Model file for the job. Use its own axes, mm. A direction names the side the tool comes from. Give positions to 0.01 mm unless a question says otherwise; leave off trailing zeros. Write each loop counter-clockwise with the first axis right and the second up, starting at its lowest first coordinate (ties: lowest second). Pieces come first, ordered by that corner, then holes. Notation, with made-up numbers: (5, 7) - (36, 7) arc R24 cw to (36, 17) - close; hole circle Ø11 at (74.5, 46). An arc over 180 degrees is marked (long way). Use CSV: the item, a comma, the result in double quotes.
from build123d import *

# Parameters (mm, degrees)
SKETCH1_R               = 61.9125
BASE_EXTRUDE_DEPTH      = 7.9248
BASE_EXTRUDE_DEPTH_BACK = 33.6677
SKETCH11_R              = 33.3375
CUT_EXTRUDE1_DEPTH      = 9.525
SKETCH12_R              = 35.7124
CUT_EXTRUDE2_DEPTH      = 2.5748
CUT_EXTRUDE2_DEPTH_BACK = 4.7752
SKETCH13_R              = 12.7
CUT_EXTRUDE3_DEPTH      = 41.0177
SKETCH32_R              = 6.7437
CUT_EXTRUDE4_DEPTH      = 45.72


with BuildPart() as part:
    # Sketch1 → Base-Extrude (new body, two sides)
    with BuildSketch(Plane(origin=(0, 0, 0), x_dir=(1, 0, 0), z_dir=(0, 1, 0))) as base_extrude_sk:
        with Locations(Location((0, 0, 0), (0, 0, 270))):  # turned: the seam where the file's is
            Circle(SKETCH1_R)
    extrude(amount=BASE_EXTRUDE_DEPTH)
    extrude(base_extrude_sk.sketch, amount=-BASE_EXTRUDE_DEPTH_BACK)

    # Sketch11 → Cut-Extrude1 (cut)
    with BuildSketch(Plane(origin=(0, 6.35, 0), x_dir=(-1, 0, 0), z_dir=(0, 1, 0))):
        with Locations(Location((0, 0, 0), (0, 0, 90))):  # turned: the seam where the file's is
            Circle(SKETCH11_R)
    extrude(amount=-CUT_EXTRUDE1_DEPTH, mode=Mode.SUBTRACT)

    # Sketch12 → Cut-Extrude2 (cut, two sides)
    with BuildSketch(Plane(origin=(0, 6.35, 0), x_dir=(-1, 0, 0), z_dir=(0, 1, 0))) as cut_extrude2_sk:
        with Locations(Location((0, 0, 0), (0, 0, 90))):  # turned: the seam where the file's is
            Circle(SKETCH12_R)
    extrude(amount=CUT_EXTRUDE2_DEPTH, mode=Mode.SUBTRACT)
    extrude(cut_extrude2_sk.sketch, amount=-CUT_EXTRUDE2_DEPTH_BACK, mode=Mode.SUBTRACT)

    # Sketch13 → Cut-Extrude3 (cut, through all)
    with BuildSketch(Plane(origin=(0, 6.35, 0), x_dir=(-1, 0, 0), z_dir=(0, 1, 0))):
        with Locations(Location((0, 0, 0), (0, 0, 90))):  # turned: the seam where the file's is
            Circle(SKETCH13_R)
    extrude(amount=-CUT_EXTRUDE3_DEPTH, mode=Mode.SUBTRACT)

    # Sketch32 → Cut-Extrude4 (cut)
    with BuildSketch(Plane(origin=(0, 7.9248, 0), x_dir=(-1, 0, 0), z_dir=(0, 1, 0))):
        with Locations(Location((0, -50.8, 0), (0, 0, 90))):  # turned: the seam where the file's is
            Circle(SKETCH32_R)
        with Locations(Location((-43.994090512, 25.4, 0), (0, 0, 90))):  # turned: the seam where the file's is
            Circle(SKETCH32_R)
        with Locations(Location((43.994090512, 25.4, 0), (0, 0, 90))):  # turned: the seam where the file's is
            Circle(SKETCH32_R)
    extrude(amount=-CUT_EXTRUDE4_DEPTH, mode=Mode.SUBTRACT)


solid = part.part
(1) Saw through at D-D, the plane y = 5. List the corners of the cut face in (x, z) (1 decimal), then the cut area to 3 significant figures.
Checked values:
outline,"circle Ø123.8 at (0, 0); hole circle Ø13.5 at (-44, 25.4); hole circle Ø71.4 at (0, 0); hole circle Ø13.5 at (0, -50.8); hole circle Ø13.5 at (44, 25.4)"
area,"7,610 mm^2"
(2) Pull direction X, two halves, no side cores. Call faces 1 (the face through (10.727, 4.705, 34.063)), 2 (the face through (1, -33.668, 13)), 3 (the face through (-60.44, -12.58, -13.42)): released by +X, released by -X, zero draft, split by the parting line, or undercut.
Checked values:
face 1,"undercut"
face 2,"zero draft"
face 3,"split by the parting line"
(3) Wall check: probe 1 along X at (y, z) = (-8, 25); probe 2 along Z at (x, y) = (-5, -17.5); probe 3 along X at (y, z) = (-16, 0). Give the ranges that are in metal, low to high. Write a range as [from, to].
Checked values:
probe 1,"x = [-56.64, -50.73], [-37.26, 37.26], [50.73, 56.64]"
probe 2,"z = [-61.71, -55.33], [-46.27, -11.67], [11.67, 61.71]"
probe 3,"x = [-61.91, -12.7], [12.7, 61.91]"
(4) Saw through at C-C, the plane z = 25.4. List the corners of the cut face in (x, y) (3 decimals).
Checked values:
outline,"(-56.462, -33.668) - (-50.738, -33.668) - (-50.738, 7.925) - (-56.462, 7.925) - close; (-37.25, -33.668) - (37.25, -33.668) - (37.25, 7.925) - (25.104, 7.925) - (25.104, 1.575) - (21.592, 1.575) - (21.592, -3.175) - (-21.592, -3.175) - (-21.592, 1.575) - (-25.104, 1.575) - (-25.104, 7.925) - (-37.25, 7.925) - close; (50.738, -33.668) - (56.462, -33.668) - (56.462, 7.925) - (50.738, 7.925) - close"
(5) 3-axis set-ups, long thin cutter, end or side, ignore diameter. For faces 4 (the face through (0.297, -12.58, -57.537)), 5 (the face through (-32, 1.575, -11)): which of +Z, -Z, +X, -X, +Y, -Y reach the whole face in a straight line?
Checked values:
face 4,"+Y, -Y"
face 5,"+Y"
(6) Saw through at A-A, the plane x = 0. List the corners of the cut face in (y, z) (1 decimal).
Checked values:
outline,"(-33.7, -61.9) - (7.9, -61.9) - (7.9, -57.5) - (-33.7, -57.5) - close; (-33.7, -44.1) - (7.9, -44.1) - (7.9, -35.7) - (1.6, -35.7) - (1.6, -33.3) - (-3.2, -33.3) - (-3.2, -12.7) - (-33.7, -12.7) - close; (-33.7, 12.7) - (-3.2, 12.7) - (-3.2, 33.3) - (1.6, 33.3) - (1.6, 35.7) - (7.9, 35.7) - (7.9, 61.9) - (-33.7, 61.9) - close"
(7) Saw through at B-B, the plane z = 0. List the corners of the cut face in (x, y) (1 decimal), then the cut area to 3 significant figures.
Checked values:
outline,"(-61.9, -33.7) - (-12.7, -33.7) - (-12.7, -3.2) - (-33.3, -3.2) - (-33.3, 1.6) - (-35.7, 1.6) - (-35.7, 7.9) - (-61.9, 7.9) - close; (12.7, -33.7) - (61.9, -33.7) - (61.9, 7.9) - (35.7, 7.9) - (35.7, 1.6) - (33.3, 1.6) - (33.3, -3.2) - (12.7, -3.2) - close"
area,"3,610 mm^2"
(8) Flat gauge pins, fed straight in: P1, Ø1.5, axis at x = -4.5, y = -22.5, coming from the -Z side; P2, Ø10, axis at y = -13, z = -20.5, coming from the +X side; P3, Ø12, axis at x = -44, y = -15, coming from the -Z side. Where does each tip first touch, or does it go through?
Checked values:
P1,"stops at z = -61.8"
P2,"stops at x = 59.94"
P3,"stops at z = -48.88"
